Geometry: final body of the model. Coordinates: model frame, mm. A direction names the side the tool comes from. Give positions to 0.01 mm unless a question says otherwise; leave off trailing zeros. Write each loop counter-clockwise with the first axis right and the second up, starting at its lowest first coordinate (ties: lowest second). Pieces come first, ordered by that corner, then holes. Notation, with made-up numbers: (33.5, -30.5) -> (42.5, -30.5) arc R32 ccw to (42.5, 1.5) -> close; hole circle Ø6 at (-38, 13). An arc over 180 degrees is marked (long way). Answer in a Markdown table with one row per item. Add a question column.
Item 1: First-contact query: P1, Ø10, axis at x = -5, y = -61, coming from the +Z side; P2, Ø6, axis at y = -81, z = -56.5, coming from the +X side (3 decimals); P3, Ø10, axis at x = -12, y = 80.5, coming from the +Z side. Flat tips, straight axial feed; report the tip coordinate or a pass-through.
Item 2: Material intervals for probe 1 along Y at (x, z) = (10, 0); probe 2 along X at (y, z) = (19.5, -82) (3 decimals); probe 3 along X at (y, z) = (98.5, -28.5) (3 decimals), sorted ascending. Write a range as from..to.
Item 3: Section query C-C on x = 22. Output: boundary loops of the cut face in (y, z).
Item 4: Draft query along X for faces 5 (the cylindrical face through (-11.5, -108.6, 14.3)), 6 (the conical face through (6.376, 100.213, 22.253)), 7 (the flat face through (-25.4, -23.3, 10.6)). Return one class per face: +X half, -X half, draft (parallel to the pull), parting line (faces both ways), or undercut.
Item 5: Access query for faces 1 (the flat face through (25.4, -23.3, -10.6)), 2 (the flat face through (15.875, 47, -23)), 3 (the cylindrical face through (-20.571, 30.911, 40.313)), 4 (the conical face through (-6.353, 100.112, 22.231)). Directions: +Z, -Z, +X, -X, +Y, -Y. A direction counts if a zero-diameter tool reaches every point of the face in a straight line with its end or side. Return the directions, or none.
Item 6: Section query D-D on x = -3.5. Output: boundary loops of the cut face in (y, z).
```python
from build123d import *

# Parameters (mm, degrees)
SKETCH2_R          = 25.4127
CUT_EXTRUDE1_DEPTH = 51.8


with BuildPart() as part:
    # Sketch1 → Revolve1 (revolve)
    with BuildSketch(Plane.XY, mode=Mode.PRIVATE) as revolve1_sk:
        with BuildLine():
            Line((-15.875, 50.8), (-15.875, 108.74375))
            ThreePointArc((-15.875, 108.74375), (-15.642516008, 109.305016008), (-15.08125, 109.5375))
            Line((-15.08125, 109.5375), (-7.9375, 109.5375))
            Line((-7.9375, 109.5375), (-6.271845407, 102.194295494))
            ThreePointArc((-6.271845407, 102.194295494), (0, 96.8375), (6.271845407, 102.194295494))
            Line((6.271845407, 102.194295494), (7.9375, 109.5375))
            Line((7.9375, 109.5375), (15.08125, 109.5375))
            ThreePointArc((15.08125, 109.5375), (15.642516008, 109.305016008), (15.875, 108.74375))
            Line((15.875, 108.74375), (15.875, 50.8))
            Line((15.875, 50.8), (25.4, 50.8))
            Line((25.4, 50.8), (25.4, 0))
            Line((25.4, 0), (-25.4, 0))
            Line((-25.4, 0), (-25.4, 50.8))
            Line((-25.4, 50.8), (-15.875, 50.8))
        make_face()
    revolve(revolve1_sk.sketch.rotate(Axis((25.4, 0, 0), (-1, 0, 0)), 90), axis=Axis((25.4, 0, 0), (-1, 0, 0)))  # turned: the seam where the file's is

    # Sketch2 → Cut-Extrude1 (cut, through all)
    with BuildSketch(Plane(origin=(25.4, 0, 0), x_dir=(0, 0, -1), z_dir=(1, 0, 0))):
        Circle(SKETCH2_R)
    extrude(amount=-CUT_EXTRUDE1_DEPTH, mode=Mode.SUBTRACT)


solid = part.part
```
Findings below:
| question | item | result |
|---|---|---|
| 1 | P1 | stops at z = 93.57 |
| 1 | P2 | stops at x = 15.875 |
| 1 | P3 | stops at z = 79.36 |
| 2 | probe 1 | y = -109.54..-25.41, 25.41..109.54 |
| 2 | probe 2 | x = -15.875..15.875 |
| 2 | probe 3 | x = -15.875..-6.35, 6.35..15.875 |
| 3 | outline | circle Ø101.6 at (0, 0); hole circle Ø50.83 at (0, 0) |
| 4 | face 5 | draft |
| 4 | face 6 | undercut |
| 4 | face 7 | -X half |
| 5 | face 1 | +Z, -Z, +X, +Y, -Y |
| 5 | face 2 | +X |
| 5 | face 3 | -X |
| 5 | face 4 | none |
| 6 | outline | circle Ø195.78 at (0, 0); hole circle Ø50.83 at (0, 0) |
